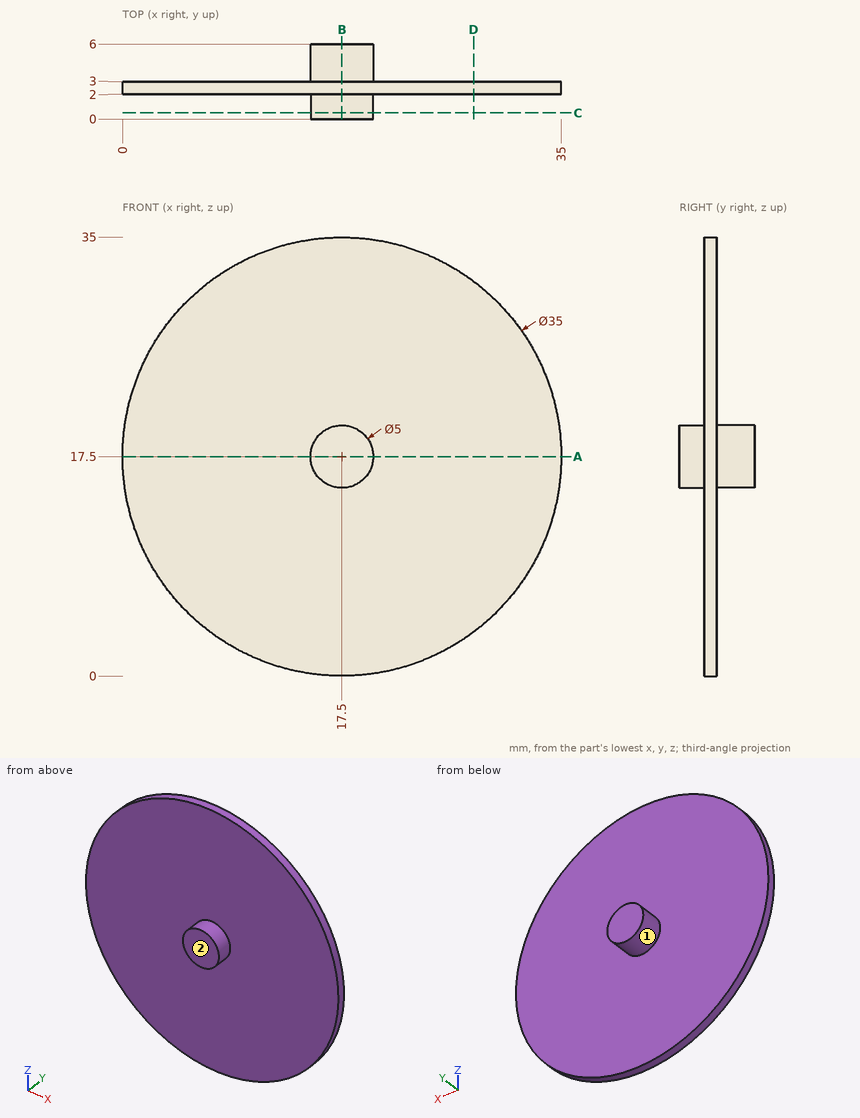
For this review, use the dimensioned drawing (mm, ordinates from the lowest corner) and the shaded views. A direction names the side the tool comes from. Round coordinates to 2 decimals unless told otherwise and drop trailing zeros. Order: outer loops, then holes, each group sorted by start corner. A loop starts at its lowest first (then second) coordinate and runs counter-clockwise, first axis right, second up. Notation, with made-up numbers: (22.5, 68.25) -> (79.5, 68.25) arc R28 cw to (79.5, 103.25) -> close; hole circle Ø10 at (62, 5.5). An arc over 180 degrees is marked (long way). Use CSV: the item, a comma, the result in double quotes. Start each with the question number.
(1) Consider section C-C on y = 0.5. Write out the cut boundary in (x, z), and give its area (3 significant figures).
(2) Wall thickness on probe 1 along Y at (x, z) = (9.5, 15.5); probe 2 along X at (y, z) = (3.55, 19); probe 3 along Z at (x, y) = (16.5, 2.5): over which ranges is each line inside the solid? List them lowest first. Write a range as from..to.
(3) Insertion check: pin 1 (1.5 mm diameter, centred on x = 23, y = 2.5, fed in from +Z); pin 2 (12 mm diameter, centred on x = 28.5, z = 15, fed in from -Y); pin 3 (1.5 mm diameter, centred on x = 29, y = 1.5, fed in from +Z). Each pin has a flat end and moves straight along its axis. Give the tip position at first contact, or say it passes through.
(4) Tool access review of the marked faces 1 and 2: name each direction out of +Z, -Z, +X, -X, +Y, -Y from which nothing blocks a thin tool from reaching the whole face with its end or side.
(5) Consider section B-B on x = 17.5. Write out the cut boundary in (y, z), and give its area (3 significant figures).
(6) Consider section D-D on x = 28. Write out the cut boundary in (y, z), and give its area (3 significant figures).
(7) Consider section A-A on z = 17.5. Write out the cut boundary in (x, y), and give its area (3 significant figures).
Responses:
1,outline,"circle Ø5 at (17.5, 17.5)"
1,area,"19.6 mm²"
2,probe 1,"2..3"
2,probe 2,"15.5..19.5"
2,probe 3,"0.03..34.97"
3,pin 1,"z = 34.34"
3,pin 2,"y = 2"
3,pin 3,"z = 31.16"
4,face 1,"+Y"
4,face 2,"+Z, -Z, +X, -X, -Y"
5,outline,"(0, 15) -> (2, 15) -> (2, 0) -> (3, 0) -> (3, 15) -> (6, 15) -> (6, 20) -> (3, 20) -> (3, 35) -> (2, 35) -> (2, 20) -> (0, 20) -> close"
5,area,"60.0 mm²"
6,outline,"(2, 3.5) -> (3, 3.5) -> (3, 31.5) -> (2, 31.5) -> close"
6,area,"28.0 mm²"
7,outline,"(0, 2) -> (15, 2) -> (15, 0) -> (20, 0) -> (20, 2) -> (35, 2) -> (35, 3) -> (20, 3) -> (20, 6) -> (15, 6) -> (15, 3) -> (0, 3) -> close"
7,area,"60.0 mm²"
